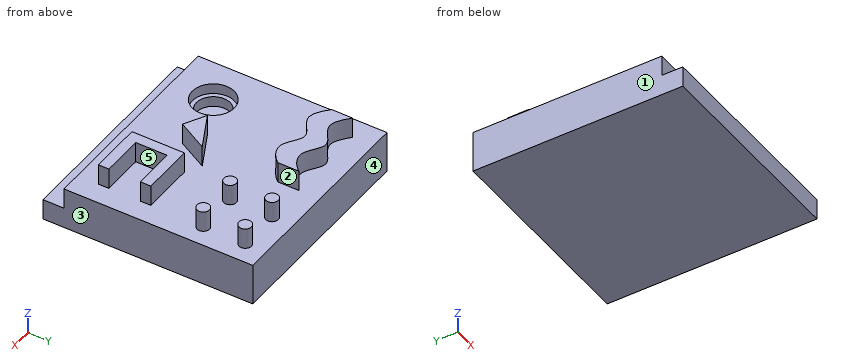
from build123d import *

# Parameters (mm, degrees)
F0_W      = 50
F0_H      = 50
F1_DEPTH  = 5
F2_W      = 50
F2_H      = 45
F3_DEPTH  = 5
F4_R      = 5
F4_R_2    = 4
F5_DEPTH  = 2.5
F6_DEPTH  = 5
F7_R      = 1.5
F8_DEPTH  = 5
F10_DEPTH = 5
F12_DEPTH = 5
F13_W     = 10
F13_H     = 2.5
F14_DEPTH = 5


with BuildPart() as f1:
    # F0 (on Top) → F1 (new body)
    with BuildSketch(Plane.XY):
        with Locations((-25, 25)):
            Rectangle(F0_W, F0_H)
    extrude(amount=F1_DEPTH)

    # F2 (on face) → F3 (join)
    with BuildSketch(Plane.XY.offset(5)):
        with Locations((-25, 27.5)):
            Rectangle(F2_W, F2_H)
    extrude(amount=F3_DEPTH)

    # F4 (on face) → F5 (cut)
    with BuildSketch(Plane.XY.offset(10)):
        with Locations((-40, 15)):
            Circle(F4_R)
        with Locations((-40, 15)):
            Circle(F4_R_2, mode=Mode.SUBTRACT)
    extrude(amount=-F5_DEPTH, mode=Mode.SUBTRACT)

    # F6 (cut): a face of the model
    f6_faces = [f1.faces().sort_by_distance(p)[0] for p in [
        (-40, 15, 10),
    ]]
    extrude(f6_faces, amount=-F6_DEPTH, mode=Mode.SUBTRACT)

    # F7 (on face) → F8 (join)
    with BuildSketch(Plane.XY.offset(10)):
        with Locations((-15, 35)):
            Circle(F7_R)
        with Locations((-5, 35)):
            Circle(F7_R)
        with Locations((-15, 45)):
            Circle(F7_R)
        with Locations((-5, 45)):
            Circle(F7_R)
    extrude(amount=F8_DEPTH)

    # F9 (on face) → F10 (join)
    with BuildSketch(Plane.XY.offset(10)):
        with BuildLine():
            add(Edge.make_bspline(
                [(-45, 45), (-43.3724021193, 43.4960327946), (-39.9998361972, 40.752966518), (-34.9419701311, 47.120567995), (-30.2322832786, 40.764761502), (-26.1633589291, 43.4685111653), (-25, 45)],
                knots=[0, 0, 0, 0, 0.25, 0.5, 0.75, 1, 1, 1, 1], degree=3))
            Line((-45, 45), (-45, 40))
            add(Edge.make_bspline(
                [(-45, 40), (-43.3724021193, 38.4960327946), (-39.9998361972, 35.752966518), (-34.9419701311, 42.120567995), (-30.2322832786, 35.764761502), (-26.1633589291, 38.4685111653), (-25, 40)],
                knots=[0, 0, 0, 0, 0.25, 0.5, 0.75, 1, 1, 1, 1], degree=3))
            Line((-25, 40), (-25, 45))
        make_face()
    extrude(amount=F10_DEPTH)

    # F11 (on face) → F12 (join)
    with BuildSketch(Plane.XY.offset(10)):
        Polygon((-21.0567055787, 24.4740903986), (-30, 20), (-24.9556113431, 17.269956793), align=None)
    extrude(amount=F12_DEPTH)

    # F13 (on face) → F14 (join)
    with BuildSketch(Plane.XY.offset(10)):
        with Locations((-10, 21.25)):
            Rectangle(F13_W, F13_H)
        Polygon((-15, 10), (-15, 12.5), (-15, 20), (-15, 22.5), (-17.5, 22.5), (-17.5, 10), align=None)
        with Locations((-10, 11.25)):
            Rectangle(F13_W, F13_H)
    extrude(amount=F14_DEPTH)


solid = f1.part
Here's how the part is built. I have some questions about the finished solid (model axes, mm). Face numbers are marked on the shaded views. A direction names the side the tool comes from. Coordinates: 2 decimals unless noted, no trailing zeros. Order: outer loops, then holes, each group sorted by start corner. A loop starts at its lowest first (then second) coordinate and runs counter-clockwise, first axis right, second up. Notation, with made-up numbers: (40, 11) -> (54, 11) arc R34 cw to (54, 43) -> close; hole circle Ø3 at (-4.75, 87). An arc over 180 degrees is marked (long way). Answer in a Markdown table with one row per item.
(1) I want a section at C-C on z = 13.5. Count the separate pieces of the cut face and the enclosed holes in it, then the cut area to 3 significant figures.
Answer key:
| item | result |
|---|---|
| separate pieces | 7 |
| enclosed holes | 0 |
| area | 233 mm^2 |
(2) On a 3-axis mill with a long thin cutter (end or side, diameter ignored), from which of +Z, -Z, +X, -X, +Y, -Y can I reach the whole of each face in a straight line? I mean the marked faces 1 and 2. Say none if no direction works.
Answer key:
| item | result |
|---|---|
| face 1 | +Z, -Z, -X, +Y, -Y |
| face 2 | +Z, +Y |
(3) Will these pins go through, and if not, where does the flat tip stop? pin 1 Ø3 at (y, z) = (21, 12.5) entering from +X; pin 2 Ø1.5 at (y, z) = (15.5, 13.5) entering from +X; pin 3 Ø5.5 at (x, z) = (-14, 13.5) entering from +Y.
Answer key:
| item | result |
|---|---|
| pin 1 | x = -5 |
| pin 2 | x = -15 |
| pin 3 | y = 46.5 |
(4) Thinking about a two-plate mould opening in Y: for the marked faces 3, 4 and 5, which applies, +Y half, -Y half, draft (parallel to the pull), parting line (faces both ways), or undercut?
Answer key:
| item | result |
|---|---|
| face 3 | draft |
| face 4 | +Y half |
| face 5 | undercut |
(5) I want a section at B-B on z = 6.5. List the corners of the cut face in (x, y) for me, then the cut area to 3 significant figures.
Answer key:
| item | result |
|---|---|
| outline | (-50, 5) -> (0, 5) -> (0, 50) -> (-50, 50) -> close; hole circle Ø8 at (-40, 15) |
| area | 2,200 mm^2 |
(6) I want a section at D-D on y = 35. List the corners of the cut face in (x, z) for me.
Answer key:
| item | result |
|---|---|
| outline | (-50, 0) -> (0, 0) -> (0, 10) -> (-3.5, 10) -> (-3.5, 15) -> (-6.5, 15) -> (-6.5, 10) -> (-13.5, 10) -> (-13.5, 15) -> (-16.5, 15) -> (-16.5, 10) -> (-50, 10) -> close |
(7) I want a section at A-A on y = 15. List the corners of the cut face in (x, z) for me.
Answer key:
| item | result |
|---|---|
| outline | (-50, 0) -> (0, 0) -> (0, 10) -> (-15, 10) -> (-15, 15) -> (-17.5, 15) -> (-17.5, 10) -> (-35, 10) -> (-35, 7.5) -> (-36, 7.5) -> (-36, 5) -> (-44, 5) -> (-44, 7.5) -> (-45, 7.5) -> (-45, 10) -> (-50, 10) -> close |
(8) Please list where these lines run through material, in increasing order: probe 1 along Y at (x, z) = (-40, 6.45); probe 2 along Y at (x, z) = (-40, 8.8); probe 3 along Z at (x, y) = (-4, 2).
Answer key:
| item | result |
|---|---|
| probe 1 | 5 to 11, 19 to 50 |
| probe 2 | 5 to 10, 20 to 50 |
| probe 3 | 0 to 5 |
